```python
from build123d import *

# Parameters (mm, degrees)
F0_R     = 22.5
F0_R_2   = 10.925
F1_DEPTH = 25.4
F2_SIZE  = 0.508
F3_SIZE  = 0.508


with BuildPart() as f1:
    # F0 (on Top) → F1 (new body)
    with BuildSketch(Plane.XY):
        Polygon((30.807892, 10.602966), (4.521396, 60.1965), (-7.053799, 60.1965), (-30.807892, 11.287956), (-30.807892, -23.549838), (-30.807892, -29.851647), (-26.064852, -29.880841), (30.927461, -29.880841), (30.807892, -27.640185), align=None)
        Circle(F0_R, mode=Mode.SUBTRACT)
        with Locations((0, 37.812808)):
            Circle(F0_R_2, mode=Mode.SUBTRACT)
    extrude(amount=F1_DEPTH)

    # F2
    f2_edges = [f1.edges().sort_by_distance(p)[0] for p in [
        (-10.925, 37.812808, 0),
    ]]
    chamfer(f2_edges, length=F2_SIZE)

    # F3
    f3_edges = [f1.edges().sort_by_distance(p)[0] for p in [
        (-10.925, 37.812808, 25.4),
    ]]
    chamfer(f3_edges, length=F3_SIZE)


solid = f1.part
```
Here's how the part is built. I have some questions about the finished solid (model axes, mm). A direction names the side the tool comes from. Coordinates: 2 decimals unless noted, no trailing zeros. Order: outer loops, then holes, each group sorted by start corner. A loop starts at its lowest first (then second) coordinate and runs counter-clockwise, first axis right, second up. Notation, with made-up numbers: M 74,15 L 104,15 A23 cw 104,30 Z; hole C 75.25,18 d3. An arc over 180 degrees is marked long. Answer as a JSON object with one key per item and string values. Group by question number.
(1) Suppose I cut it at D-D, the plane z = 17.5. State how many separate pieces and enclosed holes the cut face has, then the cut area to 3 significant figures.
(2) Suppose I cut it at B-B, the plane x = 0. Please give me the cut outline in (y, z), then the cut area to 3 significant figures.
(3) Suppose I cut it at A-A, the plane y = 0. Please give me the cut outline in (x, z).
(4) For pin 1 (12 mm diameter, centred on x = 21.5, y = 25, fed in from -Z); pin 2 (12.5 mm diameter, centred on y = -14.5, z = 8, fed in from +X); pin 3 (3 mm diameter, centred on x = -9, z = 6.5, fed in from +Y), each with a flat end and sliding along its axis, tell me the tip position at first contact or that it passes through.
(5) Which directions (+Z, -Z, +X, -X, +Y, -Y) give clear straight access to the entire face, cutting with the end or side of a thin tool? Please do faces 4 (the face through (-1, 60.196, 13)), 5 (the face through (30.808, -9, 13)).
(6) Suppose I cut it at C-C, the plane x = 17.5. Please give me the cut outline in (y, z).
(7) If we mould it in two halves opening along X, with no side actions, what happens to faces 1 (the face through (10.382, -19.961, 12.522)), 2 (the face through (0, 26, 0)), 3 (the face through (17.85, 35.05, 12.52))? For each: released by +X, released by -X, zero draft, split by the parting line, or undercut.
(8) I need wall thicknesses on probe 1 along Y at (x, z) = (0, 16.5); probe 2 along Y at (x, z) = (6.5, 13.5); probe 3 along Y at (x, z) = (16, 17). Which ranges of each line are inside material? Lowest first, please.
Values found:
{
 "1": {"separate pieces": "1", "enclosed holes": "2", "area": "2,350 mm^2"},
 "2": {"outline": "M -29.88,0 L -22.5,0 L -22.5,25.4 L -29.88,25.4 Z; M 22.5,0 L 26.38,0 L 26.89,0.51 L 26.89,24.89 L 26.38,25.4 L 22.5,25.4 Z; M 48.74,0.51 L 49.25,0 L 60.2,0 L 60.2,25.4 L 49.25,25.4 L 48.74,24.89 Z", "area": "589 mm^2"},
 "3": {"outline": "M -30.81,0 L -22.5,0 L -22.5,25.4 L -30.81,25.4 Z; M 22.5,0 L 30.81,0 L 30.81,25.4 L 22.5,25.4 Z"},
 "4": {"pin 1": "stops at z = 0", "pin 2": "stops at x = 30.81", "pin 3": "stops at y = 59.28"},
 "5": {"face 4": "+Z, -Z, +X, -X, +Y", "face 5": "+Z, -Z, +X, +Y"},
 "6": {"outline": "M -29.88,0 L -14.14,0 L -14.14,25.4 L -29.88,25.4 Z; M 14.14,0 L 35.71,0 L 35.71,25.4 L 14.14,25.4 Z"},
 "7": {"face 1": "undercut", "face 2": "zero draft", "face 3": "released by +X"},
 "8": {"probe 1": "y = -29.88 to -22.5, 22.5 to 26.89, 48.74 to 60.2", "probe 2": "y = -29.88 to -21.54, 21.54 to 29.03, 46.59 to 56.46", "probe 3": "y = -29.88 to -15.82, 15.82 to 38.54"}
}
